For this review, take the finished solid that the model builds, in its own axes (mm). Face numbers are marked on the shaded views. A direction names the side the tool comes from. Coordinates: 2 decimals unless noted, no trailing zeros. Loops run counter-clockwise (first coordinate to the right, second up) from the corner with the lowest first, then second, coordinate; pieces in that order, holes last. Notation, with made-up numbers: (68.25, 51.5) -> (112.25, 51.5) arc R20 ccw to (112.25, 59.5) -> close; hole circle Ø8 at (6.5, -26.5). An arc over 180 degrees is marked (long way). One line per item, written item: value.
from build123d import *

# Parameters (mm, degrees)
F1_DEPTH = 19.05
F2_R     = 0.79375


with BuildPart() as f1:
    # F0 (on Top) → F1 (new body)
    with BuildSketch(Plane.XY):
        with BuildLine():
            Line((-1, 6.316894), (-1, 11.958261))
            ThreePointArc((-1, 11.958261), (0, -12), (1, 11.958261))
            Line((1, 11.958261), (1, 6.316894))
            Line((1, 6.316894), (6.316894, 6.316894))
            Line((6.316894, 6.316894), (6.316894, -6.316894))
            Line((6.316894, -6.316894), (-6.316894, -6.316894))
            Line((-6.316894, -6.316894), (-6.316894, 6.316894))
            Line((-6.316894, 6.316894), (-1, 6.316894))
        make_face()
    extrude(amount=F1_DEPTH)

    # F2
    f2_edges = [f1.edges().sort_by_distance(p)[0] for p in [
        (-6.316894, 6.316894, 9.525),
        (6.316894, 6.316894, 9.525),
        (6.316894, -6.316894, 9.525),
        (-6.316894, -6.316894, 9.525),
    ]]
    fillet(f2_edges, radius=F2_R)


solid = f1.part
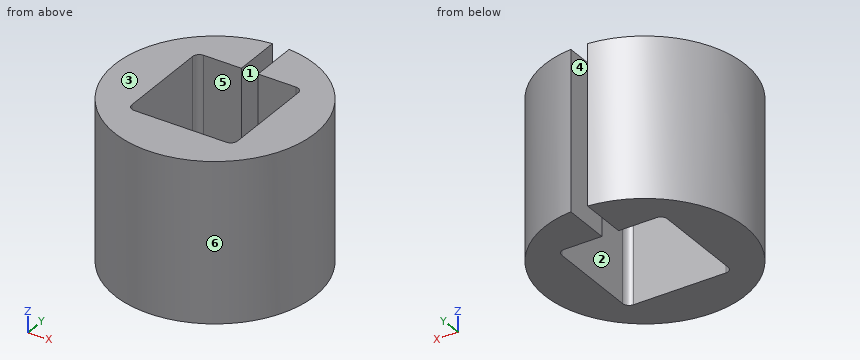
1. Take a section at D-D, the plane x = 0. Give the boundary of the cut face in (y, z).
Return value:
outline: (-12, 0) -> (-6.32, 0) -> (-6.32, 19.05) -> (-12, 19.05) -> close
2. Insertion check: pin 1 Ø10 at (y, z) = (-9.5, 14) entering from -X; pin 2 Ø1.4 at (x, z) = (3, 12.5) entering from -Y; pin 3 Ø6 at (y, z) = (5.5, 10) entering from +X. Each pin has a flat end and moves straight along its axis. Give the tip position at first contact, or say it passes through.
Return value:
pin 1: stops at x = -11.12
pin 2: stops at y = -11.78
pin 3: stops at x = 11.74
3. Take a section at C-C, the plane z = 4.75. Give the boundary of the cut face in (x, y), and give its area (3 significant figures).
Return value:
outline: (-6.32, -5.52) -> (-6.32, 5.52) arc R0.79 cw to (-5.52, 6.32) -> (-1, 6.32) -> (-1, 11.96) arc R12 ccw (long way) to (1, 11.96) -> (1, 6.32) -> (5.52, 6.32) arc R0.79 cw to (6.32, 5.52) -> (6.32, -5.52) arc R0.79 cw to (5.52, -6.32) -> (-5.52, -6.32) arc R0.79 cw to start
area: 282 mm2
4. For the marked faces 1, 2 and 3, list the 3-axis set-ups (+Z, -Z, +X, -X, +Y, -Y) from which the entire face can be reached by the end or side of a thin tool; tool diameter is ignored.
Return value:
face 1: +Z, -Z, +Y
face 2: +Z, -Z
face 3: +Z, +X, -X, +Y, -Y
5. Take a section at A-A, the plane y = 0. Give the boundary of the cut face in (x, z).
Return value:
outline: (-12, 0) -> (-6.32, 0) -> (-6.32, 19.05) -> (-12, 19.05) -> close; (6.32, 0) -> (12, 0) -> (12, 19.05) -> (6.32, 19.05) -> close
6. To check wall thickness, follow probe 1 along X at (y, z) = (4.5, 14.75); probe 2 along X at (y, z) = (5, 3.25); probe 3 along Y at (x, z) = (4, 5). State the ranges of each line that lie inside material, in increasing order. Write a range as from..to.
Return value:
probe 1: x = -11.12..-6.32, 6.32..11.12
probe 2: x = -10.91..-6.32, 6.32..10.91
probe 3: y = -11.31..-6.32, 6.32..11.31
7. Take a section at B-B, the plane x = -3.75. Give the boundary of the cut face in (y, z), and give its area (3 significant figures).
Return value:
outline: (-11.4, 0) -> (-6.32, 0) -> (-6.32, 19.05) -> (-11.4, 19.05) -> close; (6.32, 0) -> (11.4, 0) -> (11.4, 19.05) -> (6.32, 19.05) -> close
area: 194 mm2
8. The part is to be moulded in two halves that separate along Y. For the marked faces 4, 5 and 6, say which applies: pulls with the +Y half, pulls with the -Y half, needs draft (parallel to the pull), parting line crosses it, or undercut.
Return value:
face 4: needs draft
face 5: undercut
face 6: parting line crosses it
